Geometry check sheet. Reference: drawing and pictorial views, mm from the part's lowest x, y, z. Give positions to 0.01 mm unless a question says otherwise; leave off trailing zeros. Loops run counter-clockwise (first coordinate to the right, second up) from the corner with the lowest first, then second, coordinate; pieces in that order, holes last. Notation, with made-up numbers: (-32.5, -37) - (13.5, -37) arc R8 cw to (13.5, -32) - close; hole circle Ø11 at (-14.5, -28.5). An arc over 180 degrees is marked (long way). One line per question, with ' | ' between items. Start each with the question number.
1. Depth check by flat-ended pin: pin 1 Ø1 at (y, z) = (1, 7) entering from -X; pin 2 Ø2 at (x, y) = (3.5, 1) entering from -Z; pin 3 Ø1.6 at (y, z) = (1, 55) entering from +X. Enter the tip coordinate at first touch or a pass-through.
2. Mould release check, pull along X, two halves, no side actions. Record for the marked faces 1 and 2: +X half, -X half, draft (parallel to the pull), parting line (faces both ways), or undercut.
3. Section check D-D, the plane z = 34. Enter the section's corners in (x, y), then the cut area to 3 significant figures.
4. Section check B-B, the plane z = 57.65. Enter the section's corners in (x, y).
5. Thickness scan on line 1 along Z through (x, y) = (10.25, 2.3); line 2 along X through (y, z) = (2.65, 57.65); line 3 along X through (y, z) = (0.8, 57.65). Record the ranges inside material, lowest first. Write a range as from..to.
6. Section check A-A, the plane x = 99.75. Enter the section's corners in (y, z).
7. Section check C-C, the plane y = 3.4. Enter the section's corners in (x, z), then the cut area to 3 significant figures.
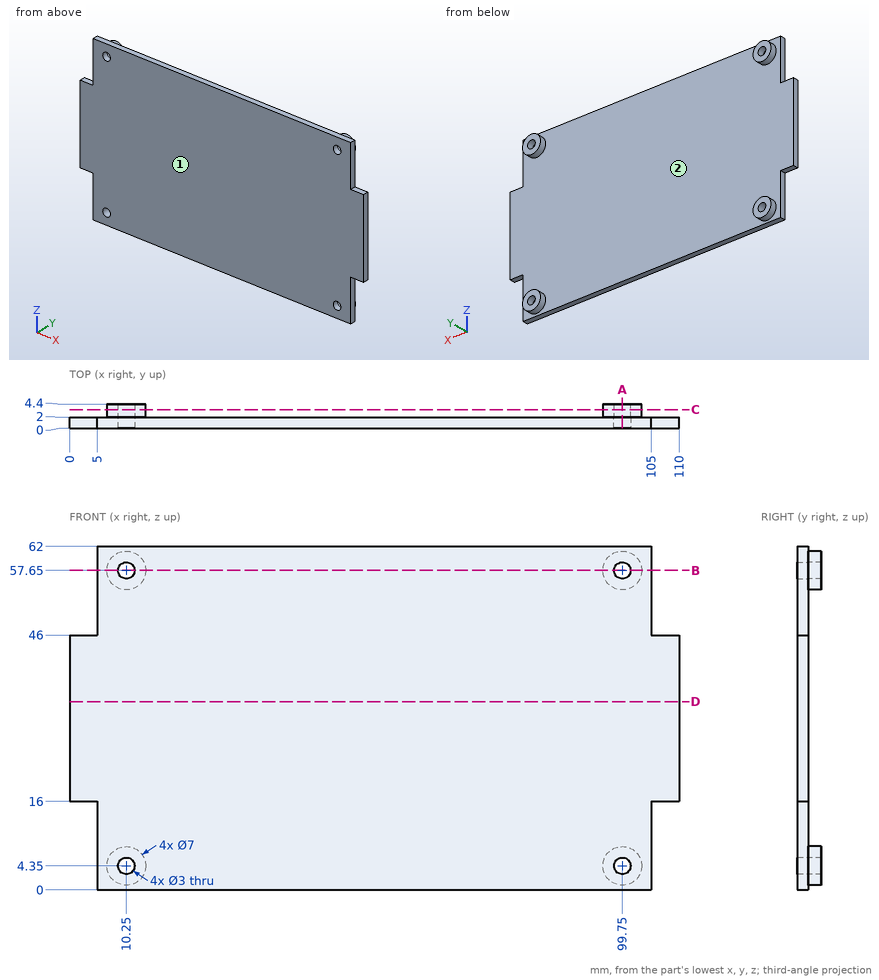
Results list:
1) pin 1: x = 5 | pin 2: z = 16 | pin 3: x = 105
2) face 1: draft | face 2: undercut
3) outline: (0, 0) - (110, 0) - (110, 2) - (0, 2) - close | area: 220 mm²
4) outline: (5, 0) - (8.75, 0) - (8.75, 4.4) - (6.75, 4.4) - (6.75, 2) - (5, 2) - close; (11.75, 0) - (98.25, 0) - (98.25, 4.4) - (96.25, 4.4) - (96.25, 2) - (13.75, 2) - (13.75, 4.4) - (11.75, 4.4) - close; (101.25, 0) - (105, 0) - (105, 2) - (103.25, 2) - (103.25, 4.4) - (101.25, 4.4) - close
5) line 1: 0.85..2.85, 5.85..7.85, 54.15..56.15, 59.15..61.15 | line 2: 6.75..8.75, 11.75..13.75, 96.25..98.25, 101.25..103.25 | line 3: 5..8.75, 11.75..98.25, 101.25..105
6) outline: (0, 0) - (2, 0) - (2, 0.85) - (4.4, 0.85) - (4.4, 2.85) - (0, 2.85) - close; (0, 5.85) - (4.4, 5.85) - (4.4, 7.85) - (2, 7.85) - (2, 54.15) - (4.4, 54.15) - (4.4, 56.15) - (0, 56.15) - close; (0, 59.15) - (4.4, 59.15) - (4.4, 61.15) - (2, 61.15) - (2, 62) - (0, 62) - close
7) outline: circle Ø7 at (10.25, 4.35); circle Ø7 at (10.25, 57.65); circle Ø7 at (99.75, 4.35); circle Ø7 at (99.75, 57.65); hole circle Ø3 at (10.25, 4.35); hole circle Ø3 at (10.25, 57.65); hole circle Ø3 at (99.75, 4.35); hole circle Ø3 at (99.75, 57.65) | area: 126 mm²
